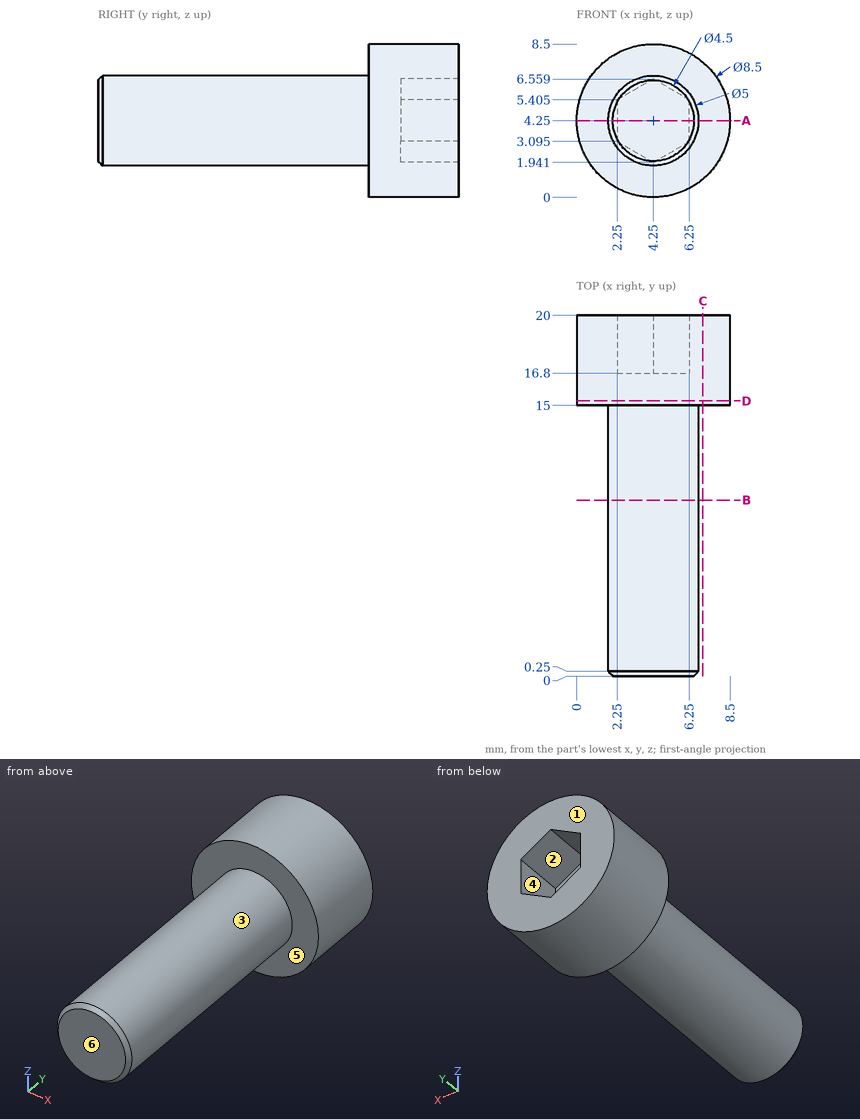
For this review, use the dimensioned drawing (mm, ordinates from the lowest corner) and the shaded views. A direction names the side the tool comes from. Round coordinates to 2 decimals unless told otherwise and drop trailing zeros. Write each loop counter-clockwise with the first axis right and the second up, starting at its lowest first coordinate (ties: lowest second). Pieces come first, ordered by that corner, then holes. Notation, with made-up numbers: (6.5, 67.25) -> (46.5, 67.25) arc R19 cw to (46.5, 98.25) -> close; hole circle Ø4 at (82, 63.25). An arc over 180 degrees is marked (long way). Use one line per item in the form item = value.
Q1. Machinability: for the marked faces 4, 5 and 6, which of the approach directions +Z, -Z, +X, -X, +Y, -Y give a long, thin tool a straight path to every point of the face, cutting with its end or side? Answer none if there is none.
Resolved:
face_4 = +Y
face_5 = -Y
face_6 = +Z, -Z, +X, -X, -Y
Q2. The part is to be moulded in two halves that separate along X. For the marked faces 1, 2 and 3, say which applies: released by +X, released by -X, zero draft, split by the parting line, or undercut.
Resolved:
face_1 = zero draft
face_2 = undercut
face_3 = split by the parting line
Q3. Consider section A-A (z = 4.25). State the section outline as (x, y) points, then the cut area to 3 significant figures.
Resolved:
outline = (0, 15) -> (1.75, 15) -> (1.75, 0.25) -> (2, 0) -> (6.5, 0) -> (6.75, 0.25) -> (6.75, 15) -> (8.5, 15) -> (8.5, 20) -> (6.25, 20) -> (6.25, 16.8) -> (2.25, 16.8) -> (2.25, 20) -> (0, 20) -> close
area = 105 mm²
Q4. To check wall thickness, follow probe 1 along X at (y, z) = (15.75, 8); probe 2 along Y at (x, z) = (3.5, 4.75); probe 3 along Y at (x, z) = (2.75, 7.75). State the ranges of each line that lie inside material, in increasing order. Write a range as from..to.
Resolved:
probe_1 = 2.25..6.25
probe_2 = 0..16.8
probe_3 = 15..20
Q5. Consider section D-D (y = 15.25). State the section outline as (x, z) points.
Resolved:
outline = circle Ø8.5 at (4.25, 4.25)
Q6. Consider section C-C (x = 7). State the section outline as (y, z) points.
Resolved:
outline = (15, 1.01) -> (20, 1.01) -> (20, 7.49) -> (15, 7.49) -> close
Q7. Consider section B-B (y = 9.75). State the section outline as (x, z) points.
Resolved:
outline = circle Ø5 at (4.25, 4.25)
Q8. Clearance check with flat-ended pins moving along their axes: pin 1 Ø1.5 at (x, y) = (5, 7.5) entering from +Z; pin 2 Ø1.5 at (x, y) = (2, 11) entering from +Z; pin 3 Ø1 at (y, z) = (4.5, 6.5) entering from -X (1 decimal). State where each tip first meets the part, or that it passes through.
Resolved:
pin_1 = 6.75
pin_2 = 6.25
pin_3 = 2.5
